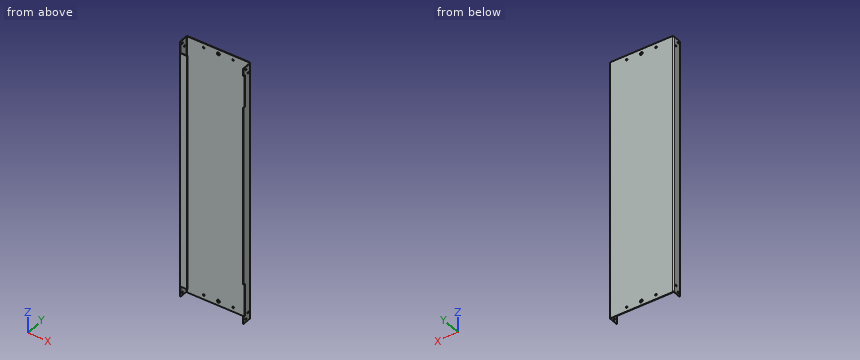
from build123d import *

# Parameters (mm, degrees)
SM_BASE_FLANGE_1_DEPTH = 398.5
SKETCH_6_W             = 1.5
SKETCH_6_H             = 30
CUT_EXTRUDE_1_DEPTH    = 3
SKETCH_7_W             = 23.5
SKETCH_7_H             = 35.5
CUT_EXTRUDE_2_DEPTH    = 3
SKETCH_8_R             = 2.5
CUT_EXTRUDE_3_DEPTH    = 446.104762949
SKETCH_10_R            = 2.5
SKETCH_10_R_2          = 4.5
CUT_EXTRUDE_4_DEPTH    = 10
SKETCH_11_W            = 100
SKETCH_11_H            = 7
CUT_EXTRUDE_2108_DEPTH = 10


# Sheet-metal steps are written as plain solids
with BuildPart() as part:
    # Sketch 1 → Базовая кромка1 (new, symmetric)
    with BuildSketch(Plane.XY):
        with BuildLine():
            Line((-74.5, -30), (-95, -30))
            ThreePointArc((-95, -30), (-97.121320344, -29.121320344), (-98, -27))
            Line((-98, -27), (-98, -3))
            ThreePointArc((-98, -3), (-97.121320344, -0.878679656), (-95, 0))
            Line((-95, 0), (95, 0))
            ThreePointArc((95, 0), (97.121320344, -0.878679656), (98, -3))
            Line((98, -3), (98, -30))
            Line((98, -30), (96.5, -30))
            Line((96.5, -30), (96.5, -3))
            ThreePointArc((96.5, -3), (96.060660172, -1.939339828), (95, -1.5))
            Line((95, -1.5), (-95, -1.5))
            ThreePointArc((-95, -1.5), (-96.060660172, -1.939339828), (-96.5, -3))
            Line((-96.5, -3), (-96.5, -27))
            ThreePointArc((-96.5, -27), (-96.060660172, -28.060660172), (-95, -28.5))
            Line((-95, -28.5), (-74.5, -28.5))
            Line((-74.5, -28.5), (-74.5, -30))
        make_face()
    extrude(amount=SM_BASE_FLANGE_1_DEPTH, both=True)

    # Эскиз6 → Вырез-Вытянуть1 (cut)
    with BuildSketch(Plane.ZY.offset(98)):
        with Locations((397.75, -15)):
            Rectangle(SKETCH_6_W, SKETCH_6_H)
        with Locations((-397.75, -15)):
            Rectangle(SKETCH_6_W, SKETCH_6_H)
    cut_extrude_1 = extrude(amount=-CUT_EXTRUDE_1_DEPTH, mode=Mode.SUBTRACT)

    # Зеркальное отражение1: Вырез-Вытянуть1 across plane
    add(cut_extrude_1.mirror(Plane(origin=(0, 0, 0), x_dir=(0, 0, 1), z_dir=(1, 0, 0))), mode=Mode.SUBTRACT)

    # Эскиз7 → Вырез-Вытянуть2 (cut)
    with BuildSketch(Plane.XZ.offset(30)):
        with Locations((-86.25, 380.75)):
            Rectangle(SKETCH_7_W, SKETCH_7_H)
        with Locations((-86.25, -380.75)):
            Rectangle(SKETCH_7_W, SKETCH_7_H)
    extrude(amount=-CUT_EXTRUDE_2_DEPTH, mode=Mode.SUBTRACT)

    # Эскиз8 → Вырез-Вытянуть3 (cut, through all)
    with BuildSketch(Plane.ZY.offset(98)):
        with Locations((-388, -20)):
            Circle(SKETCH_8_R)
        with Locations((-373, -10)):
            Circle(SKETCH_8_R)
        with Locations(Location((373, -10, 0), (0, 0, 180))):
            Circle(SKETCH_8_R)
        with Locations(Location((388, -20, 0), (0, 0, 180))):
            Circle(SKETCH_8_R)
    extrude(amount=-CUT_EXTRUDE_3_DEPTH, mode=Mode.SUBTRACT)

    # Эскиз10 → Вырез-Вытянуть4 (cut)
    with BuildSketch(Plane(origin=(0, 0, 0), x_dir=(1, 0, 0), z_dir=(0, 1, 0))):
        with Locations(Location((-44.25, -385, 0), (0, 0, 270))):
            Circle(SKETCH_10_R)
        with Locations(Location((0.75, -385, 0), (0, 0, 270))):
            Circle(SKETCH_10_R_2)
        with Locations(Location((45.75, -385, 0), (0, 0, 270))):
            Circle(SKETCH_10_R)
        with Locations(Location((45.75, 385, 0), (0, 0, 90))):
            Circle(SKETCH_10_R)
        with Locations(Location((0.75, 385, 0), (0, 0, 90))):
            Circle(SKETCH_10_R_2)
        with Locations(Location((-44.25, 385, 0), (0, 0, 90))):
            Circle(SKETCH_10_R)
    extrude(amount=-CUT_EXTRUDE_4_DEPTH, mode=Mode.SUBTRACT)

    # Эскиз11 → Cut-Extrude 2108 (cut)
    with BuildSketch(Plane(origin=(98, 0, 0), x_dir=(0, 0, -1), z_dir=(1, 0, 0))):
        with Locations((325, -26.5)):
            Rectangle(SKETCH_11_W, SKETCH_11_H)
        with Locations((-325, -26.5)):
            Rectangle(SKETCH_11_W, SKETCH_11_H)
    extrude(amount=-CUT_EXTRUDE_2108_DEPTH, mode=Mode.SUBTRACT)


solid = part.part
Geometry: final body of the model. Coordinates: model frame, mm. Give positions to 0.01 mm unless a question says otherwise; leave off trailing zeros. Loops run counter-clockwise (first coordinate to the right, second up) from the corner with the lowest first, then second, coordinate; pieces in that order, holes last. Notation, with made-up numbers: (79.25, -2.5) -> (137.25, -2.5) arc R14 cw to (137.25, 12.5) -> close; hole circle Ø10 at (78.25, -7). An arc over 180 degrees is marked (long way). Put each result on its own line as item: value.
1. Pin query (flat end, axial travel): P1, Ø3, axis at y = -10, z = 373, coming from the -X side; P2, Ø3, axis at x = -71.5, z = 187.5, coming from the -Y side; P3, Ø1.2, axis at y = -0.5, z = 398, coming from the -X side; P4, Ø2.5, axis at x = -97, y = -10.5, coming from the -Z side. Return the tip coordinate at first contact, or that it passes through.
Taken from the geometry:
P1: passes through
P2: stops at y = -1.5
P3: stops at x = -95
P4: stops at z = -397
2. Ray query, line 1 along Y through (x, z) = (-75.5, 301); line 2 along X through (y, z) = (-15.5, -243); line 3 along Y through (x, z) = (-9, -166). Return the intervals inside material, ascending. Write a range as [from, to].
Taken from the geometry:
line 1: y = [-30, -28.5], [-1.5, 0]
line 2: x = [-98, -96.5], [96.5, 98]
line 3: y = [-1.5, 0]
3. Cut plane C-C (z = -39.5). Return the cut outline in (x, y), plus the area to 3 significant figures.
Taken from the geometry:
outline: (-98, -27) arc R3 ccw to (-95, -30) -> (-74.5, -30) -> (-74.5, -28.5) -> (-95, -28.5) arc R1.5 cw to (-96.5, -27) -> (-96.5, -3) arc R1.5 cw to (-95, -1.5) -> (95, -1.5) arc R1.5 cw to (96.5, -3) -> (96.5, -30) -> (98, -30) -> (98, -3) arc R3 ccw to (95, 0) -> (-95, 0) arc R3 ccw to (-98, -3) -> close
area: 408 mm2
4. Cut plane A-A (z = 327). Return the cut outline in (x, y), plus the area to 3 significant figures.
Taken from the geometry:
outline: (-98, -27) arc R3 ccw to (-95, -30) -> (-74.5, -30) -> (-74.5, -28.5) -> (-95, -28.5) arc R1.5 cw to (-96.5, -27) -> (-96.5, -3) arc R1.5 cw to (-95, -1.5) -> (95, -1.5) arc R1.5 cw to (96.5, -3) -> (96.5, -23) -> (98, -23) -> (98, -3) arc R3 ccw to (95, 0) -> (-95, 0) arc R3 ccw to (-98, -3) -> close
area: 398 mm2
5. Cut plane B-B (x = -27). Return the cut outline in (y, z), plus the area to 3 significant figures.
Taken from the geometry:
outline: (-1.5, -398.5) -> (0, -398.5) -> (0, 398.5) -> (-1.5, 398.5) -> close
area: 1,200 mm2
